from build123d import *

# Parameters (mm, degrees)
BOSS_EXTRUDE1_DEPTH = 3.175
FILLET1_R           = 12.7
SKETCH2_R           = 1.5875
CUT_EXTRUDE1_DEPTH  = 315.453256661


with BuildPart() as part:
    # Sketch1 → Boss-Extrude1 (new body)
    with BuildSketch(Plane(origin=(0, 0, 0), x_dir=(1, 0, 0), z_dir=(0, 1, 0))):
        with BuildLine():
            Line((0, 228.6), (0, 127))
            Line((0, 127), (85.952954744, 127))
            ThreePointArc((85.952954744, 127), (107.95, 139.7), (129.947045256, 127))
            Line((129.947045256, 127), (215.9, 127))
            Line((215.9, 127), (215.9, 228.6))
            Line((215.9, 228.6), (0, 228.6))
        make_face()
    extrude(amount=BOSS_EXTRUDE1_DEPTH)

    # Fillet1
    fillet1_edges = [part.edges().sort_by_distance(p)[0] for p in [
        (85.952954744, 1.5875, -127),
        (129.947045256, 1.5875, -127),
    ]]
    fillet(fillet1_edges, radius=FILLET1_R)

    # Sketch2 → Cut-Extrude1 (cut, through all)
    with BuildSketch(Plane(origin=(0, 3.175, 0), x_dir=(1, 0, 0), z_dir=(0, 1, 0))):
        with Locations(Location((6.35, 146.05, 0), (0, 0, 270))):
            Circle(SKETCH2_R)
        with Locations(Location((57.15, 222.25, 0), (0, 0, 270))):
            Circle(SKETCH2_R)
        with Locations(Location((158.75, 222.25, 0), (0, 0, 270))):
            Circle(SKETCH2_R)
        with Locations(Location((209.55, 146.05, 0), (0, 0, 270))):
            Circle(SKETCH2_R)
    extrude(amount=-CUT_EXTRUDE1_DEPTH, mode=Mode.SUBTRACT)


solid = part.part
The listing builds one solid part. Answer for the finished solid, in the listing's coordinates (mm). A direction names the side the tool comes from. Give positions to 0.01 mm unless a question says otherwise; leave off trailing zeros. Loops run counter-clockwise (first coordinate to the right, second up) from the corner with the lowest first, then second, coordinate; pieces in that order, holes last. Notation, with made-up numbers: (-34, 45.25) - (16, 45.25) arc R30 ccw to (16, 83.25) - close; hole circle Ø5 at (-8, -29.75). An arc over 180 degrees is marked (long way). Answer as a JSON object with one key per item and string values.
1. Find the intervals of material crossed by L1, parallel to X at y = 0.7, z = -222.25; L2, parallel to X at y = 2.25, z = -146.05; L3, parallel to Z at x = 209.55, y = 1.3, in increasing order. Write a range as [from, to].
Determined:
{"L1": "[0, 55.56], [58.74, 157.16], [160.34, 215.9]", "L2": "[0, 4.76], [7.94, 207.96], [211.14, 215.9]", "L3": "[-228.6, -147.64], [-144.46, -127]"}
2. For a pull along X with two mould halves and no side action, classify faces 3 (the cylindrical face through (84.668, 1.61, -128.076)), 4 (the flat face through (106, 0, -179)) as pulls with the +X half, pulls with the -X half, needs draft (parallel to the pull), parting line crosses it, or undercut.
Determined:
{"face 3": "undercut", "face 4": "needs draft"}
3. A cutting plane is placed at C-C (x = 121). Write down the section's boundary in (y, z) (3 decimals), then the cut area to 3 significant figures.
Determined:
{"outline": "(0, -228.6) - (3.175, -228.6) - (3.175, -136.091) - (0, -136.091) - close", "area": "294 mm²"}
4. A cutting plane is placed at B-B (x = 94.5). Write down the section's boundary in (y, z) (3 decimals), then the cut area to 3 significant figures.
Determined:
{"outline": "(0, -228.6) - (3.175, -228.6) - (3.175, -135.847) - (0, -135.847) - close", "area": "294 mm²"}
5. For faces 1 (the cylindrical face through (131.095, 1.61, -128.137)), 2 (the flat face through (106, 3.175, -179)), determine the directions among +Z, -Z, +X, -X, +Y, -Y from which every point of the face is accessible in a straight line to the end or side of a thin tool.
Determined:
{"face 1": "+Z, +Y, -Y", "face 2": "+Z, -Z, +X, -X, +Y"}
6. A cutting plane is placed at A-A (y = 1.15). Give the number of separate pieces and of enclosed holes in the cut face, then the cut area to 3 significant figures.
Determined:
{"separate pieces": "1", "enclosed holes": "4", "area": "21,500 mm²"}
